Input: part model. Units: mm. Frame: model coordinates. A direction names the side the tool comes from. Coordinates: 2 decimals unless noted, no trailing zeros. Write each loop counter-clockwise with the first axis right and the second up, starting at its lowest first coordinate (ties: lowest second). Pieces come first, ordered by that corner, then holes.
from build123d import *

# Parameters (mm, degrees)
SKETCH_R      = 1.6
PAD_DEPTH     = 2
SKETCH001_R   = 5.5
SKETCH001_R_2 = 1.6
PAD001_DEPTH  = 0.5
SKETCH002_R   = 3.75
SKETCH002_R_2 = 1.6
PAD002_DEPTH  = 3.5


with BuildPart() as part:
    # Sketch → Pad (new body)
    with BuildSketch(Plane.XY):
        with BuildLine():
            ThreePointArc((-27, 0), (-45.523309, 11.768307), (-48.306624, -10))
            Line((-48.306624, -13), (-48.306624, -10))
            Line((-27.5, -13), (-48.306624, -13))
            Line((-27.5, -10), (-27.5, -13))
            Line((-27.5, -10), (27.5, -10))
            Line((27.5, -10), (27.5, -13))
            Line((27.5, -13), (48.306624, -13))
            Line((48.306624, -13), (48.306624, -10))
            ThreePointArc((48.306624, -10), (45.523309, 11.768307), (27, 0))
            Line((-27, 0), (27, 0))
        make_face()
        with Locations((-40, 0)):
            Circle(SKETCH_R, mode=Mode.SUBTRACT)
        with Locations((40, 0)):
            Circle(SKETCH_R, mode=Mode.SUBTRACT)
    extrude(amount=PAD_DEPTH)

    # Sketch001 → Pad001 (new body)
    with BuildSketch(Plane.XY.offset(2)):
        with Locations((-40, 0)):
            Circle(SKETCH001_R)
        with Locations((-40, 0)):
            Circle(SKETCH001_R_2, mode=Mode.SUBTRACT)
        with Locations((40, 0)):
            Circle(SKETCH001_R)
        with Locations((40, 0)):
            Circle(SKETCH001_R_2, mode=Mode.SUBTRACT)
    extrude(amount=PAD001_DEPTH)

    # Sketch002 → Pad002 (new body)
    with BuildSketch(Plane.XY.offset(2.5)):
        with Locations((-40, 0)):
            Circle(SKETCH002_R)
        with Locations((-40, 0)):
            Circle(SKETCH002_R_2, mode=Mode.SUBTRACT)
        with Locations((40, 0)):
            Circle(SKETCH002_R)
        with Locations((40, 0)):
            Circle(SKETCH002_R_2, mode=Mode.SUBTRACT)
    extrude(amount=PAD002_DEPTH)


solid = part.part
Item 1: Material intervals for line 1 (X direction, y = -0.25, z = 2.95); line 2 (X direction, y = -1.25, z = 5.55); line 3 (Y direction, x = 40, z = 1.65), sorted ascending.
Item 2: Pin query (flat end, axial travel): pin 1 Ø2 at (y, z) = (-11.5, 1) entering from -X; pin 2 Ø13 at (x, y) = (11.5, -2.5) entering from +Z; pin 3 Ø1.6 at (y, z) = (-11.5, 0.5) entering from +X; pin 4 Ø3 at (x, y) = (40, 0) entering from -Z. Return the tip coordinate at first contact, or that it passes through.
Item 3: Access query for faces 1 (the face through (44, -1, 2.5)), 2 (the face through (0, -10, 1)), 3 (the face through (48.307, -12, 1)). Directions: +Z, -Z, +X, -X, +Y, -Y. A direction counts if a zero-diameter tool reaches every point of the face in a straight line with its end or side. Return the directions, or none.
Item 4: Section query C-C, the plane x = 16. Return loops of the section in (y, z).
Item 5: Section query B-B, the plane z = 3.8. Return loops of the section in (x, y).
Item 6: Pull-direction query (X, two-part tool) for faces 4 (the face through (36.254, 0.165, 4.226)), 5 (the face through (-1, -3, 0)), 6 (the face through (-48.307, -12, 1)); classes: released by +X, released by -X, zero draft, split by the parting line, or undercut.
Item 7: Section query A-A, the plane x = 40. Return loops of the section in (y, z).
The answers:
1. line 1: x = -43.74 to -41.58, -38.42 to -36.26, 36.26 to 38.42, 41.58 to 43.74
1. line 2: x = -43.54 to -41, -39 to -36.46, 36.46 to 39, 41 to 43.54
1. line 3: y = -13 to -1.6, 1.6 to 13
2. pin 1: stops at x = -48.31
2. pin 2: stops at z = 2
2. pin 3: stops at x = 48.31
2. pin 4: passes through
3. face 1: +Z
3. face 2: +Z, -Z, -Y
3. face 3: +Z, -Z, +X, -Y
4. outline: (-10, 0) - (0, 0) - (0, 2) - (-10, 2) - close
5. outline: circle Ø7.5 at (-40, 0); circle Ø7.5 at (40, 0); hole circle Ø3.2 at (-40, 0); hole circle Ø3.2 at (40, 0)
6. face 4: undercut
6. face 5: zero draft
6. face 6: released by -X
7. outline: (-13, 0) - (-1.6, 0) - (-1.6, 6) - (-3.75, 6) - (-3.75, 2.5) - (-5.5, 2.5) - (-5.5, 2) - (-13, 2) - close; (1.6, 0) - (13, 0) - (13, 2) - (5.5, 2) - (5.5, 2.5) - (3.75, 2.5) - (3.75, 6) - (1.6, 6) - close
